The model under review builds one solid part; all positions refer to its coordinate system, in mm. Face numbers are marked on the shaded views. Round coordinates to 2 decimals unless told otherwise and drop trailing zeros. Write each loop counter-clockwise with the first axis right and the second up, starting at its lowest first coordinate (ties: lowest second). Pieces come first, ordered by that corner, then holes. Notation, with made-up numbers: (66, 10) - (124, 10) arc R15 ccw to (124, 32) - close; hole circle Ø6 at (57, -34). An arc over 180 degrees is marked (long way). Write each question's results on one line, items separated by ' | '.
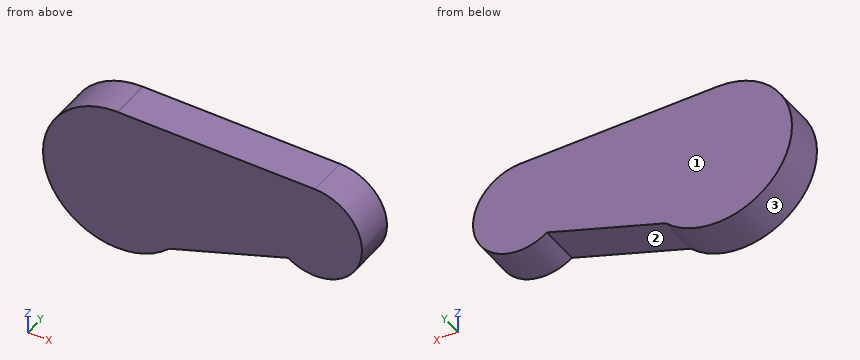
```python
from build123d import *

# Parameters (mm, degrees)
F1_DEPTH = 38.1


with BuildPart() as f1:
    # F0 (on Front) → F1 (new body)
    with BuildSketch(Plane.XZ):
        with BuildLine():
            ThreePointArc((-48.564447, -60.954478), (-54.078042, -88.154653), (-69.748399, -111.060748))
            Line((-69.748399, -111.060748), (41.969208, -73.256539))
            ThreePointArc((41.969208, -73.256539), (24.58164, -23.316982), (67.255602, 7.911527))
            Line((67.255602, 7.911527), (-117.735768, 8.892225))
            ThreePointArc((-117.735768, 8.892225), (-68.783669, -11.803604), (-48.564447, -60.954478))
        make_face()
        with BuildLine():
            Line((-117.735768, 8.892225), (-118.352549, 8.895495))
            ThreePointArc((-118.352549, 8.895495), (-183.152212, -87.185076), (-69.748399, -111.060748))
            ThreePointArc((-69.748399, -111.060748), (-54.078042, -88.154653), (-48.564447, -60.954478))
            ThreePointArc((-48.564447, -60.954478), (-68.783669, -11.803604), (-117.735768, 8.892225))
        make_face()
        with BuildLine():
            ThreePointArc((67.255602, 7.911527), (24.58164, -23.316982), (41.969208, -73.256539))
            ThreePointArc((41.969208, -73.256539), (87.784071, -75.839938), (111.469962, -36.537848))
            ThreePointArc((111.469962, -36.537848), (98.53406, -5.190374), (67.255602, 7.911527))
        make_face()
    extrude(amount=F1_DEPTH)


solid = f1.part
```
Q1. The part is to be moulded in two halves that separate along X. For the marked faces 1, 2 and 3, say which applies: released by +X, released by -X, zero draft, split by the parting line, or undercut.
Evaluation:
face 1: zero draft | face 2: undercut | face 3: split by the parting line
Q2. Insertion check: P1, Ø3, axis at x = -0.5, y = -13, coming from the -Z side; P2, Ø1.5, axis at x = -0.5, y = -16.5, coming from the +Z side; P3, Ø1, axis at x = -51.5, y = -26.5, coming from the -Z side. Each pin has a flat end and moves straight along its axis. Give the tip position at first contact, or say it passes through.
Evaluation:
P1: stops at z = -88.14 | P2: stops at z = 8.27 | P3: stops at z = -105.05
Q3. For probe 1 along Z at (x, y) = (66.5, -21.5); probe 2 along X at (y, z) = (-37, -62.5); probe 3 along Z at (x, y) = (61.5, -16), list the stretches that pass through material, from the lowest coordinate up.
Evaluation:
probe 1: z = -80.98 to 7.92 | probe 2: x = -188.25 to 103.1 | probe 3: z = -80.64 to 7.94
Q4. We need section B-B (z = -88.5). State the section outline as (x, y) points, plus the area to 3 significant figures.
Evaluation:
outline: (-182.6, -38.1) - (-3.08, -38.1) - (-3.08, 0) - (-182.6, 0) - close | area: 6,840 mm^2
Q5. We need section C-C (x = -15). State the section outline as (y, z) points.
Evaluation:
outline: (-38.1, -92.53) - (0, -92.53) - (0, 8.35) - (-38.1, 8.35) - close
Q6. We need section A-A (y = -19). State the section outline as (x, z) points, plus the area to 3 significant figures.
Evaluation:
outline: (-118.35, 8.9) arc R69.85 ccw (long way) to (-69.75, -111.06) - (41.97, -73.26) arc R44.45 ccw to (111.47, -36.54) arc R44.45 ccw to (67.26, 7.91) - (-117.74, 8.89) - close | area: 30,700 mm^2
